Source: CAD feature listing. Evaluate the final solid. Frame: model axes, mm. A direction names the side the tool comes from. Round coordinates to 2 decimals unless told otherwise and drop trailing zeros. Loops run counter-clockwise (first coordinate to the right, second up) from the corner with the lowest first, then second, coordinate; pieces in that order, holes last.
(1) Section A-A, the plane y = 5. Return the cut outline in (x, z), plus the area to 3 significant figures.
(2) Section D-D, the plane y = 38. Return the cut outline in (x, z).
(3) Mould query, pull axis Z, two halves, no side actions, for faces 6 (the flat face through (35, 60, 10)), 7 (the cylindrical face through (62, 12, 0)), 8 (the cylindrical face through (0, 83, -31)). Classes: pulls with the +Z half, pulls with the -Z half, needs draft (parallel to the pull), parting line crosses it, or undercut.
(4) First-contact query: pin 1 Ø5 at (x, y) = (31, 66.5) entering from +Z; pin 2 Ø22 at (x, y) = (-76, 18) entering from +Z; pin 3 Ø13 at (x, z) = (-34.5, 5.5) entering from +Y. Flat tips, straight axial feed; report the tip coordinate or a pass-through.
(5) Set-up query: faces 1 (the flat face through (-80, 12, 8)), 2 (the flat face through (-51.439, 12.325, 37.566)), 3 (the flat face through (80, 12, -8)), 4 (the cylindrical face through (0, 4, 52)), 5 (the flat face through (12, 80, 28)). Return all of +Z, -Z, +X, -X, +Y, -Y with unobstructed straight access to the full face (end or side cutting, diameter ignored); none if empty.
(6) Section C-C, the plane x = 11.5. Return the cut outline in (y, z), plus the area to 3 significant figures.
(7) Section B-B, the plane z = 0. Return the cut outline in (x, y), plus the area to 3 significant figures.
(8) Material intervals for probe 1 along Y at (x, z) = (24, 0); probe 2 along X at (y, z) = (69.5, -4); probe 3 along X at (y, z) = (38.5, 50), sorted ascending.
```python
from build123d import *
from build123d.topology import SkipClean

# Parameters (mm, degrees)
EXTRUDE_1_DEPTH          = 25
SKETCH_2_R               = 45
EXTRUDE_2_DEPTH          = 60
SKETCH_3_R               = 38
CUT_EXTRUDE_1_DEPTH      = 5
SKETCH_4_R               = 24
CUT_EXTRUDE_2_DEPTH      = 132.164019457
CUT_EXTRUDE_3_DEPTH      = 121.016665509
SKETCH_7_W               = 96.437930536
SKETCH_7_H               = 64.787813211
CUT_EXTRUDE_4_DEPTH      = 132.164019457
SKETCH_8_R               = 4
CUT_EXTRUDE_5_DEPTH      = 156.20953579
EXTRUDE_3_REACH          = 158.045
SKETCH_9_R               = 30
CUT_EXTRUDE_6_REACH      = 158.045
CUT_EXTRUDE_6_END_RADIUS = 24
SKETCH_10_R              = 20


with BuildPart() as part:
    # 草图1 → 凸台-拉伸1 (new body)
    with BuildSketch(Plane(origin=(0, 0, 0), x_dir=(1, 0, 0), z_dir=(0, 1, 0))):
        with BuildLine():
            Line((-90, 38), (90, 38))
            Line((90, 38), (90, 8))
            Line((90, 8), (70, 8))
            ThreePointArc((70, 8), (62, 0), (70, -8))
            Line((70, -8), (90, -8))
            Line((90, -8), (90, -25))
            Line((90, -25), (13.942908677, -49.785456613))
            ThreePointArc((13.942908677, -49.785456613), (0, -52), (-13.942908677, -49.785456613))
            Line((-13.942908677, -49.785456613), (-90, -25))
            Line((-90, -25), (-90, -8))
            Line((-90, -8), (-70, -8))
            ThreePointArc((-70, -8), (-62, 0), (-70, 8))
            Line((-70, 8), (-90, 8))
            Line((-90, 8), (-90, 38))
        make_face()
    extrude(amount=EXTRUDE_1_DEPTH)

    # 草图2 → 凸台-拉伸2 (add)
    with SkipClean():  # the faces are left unmerged after this step: merging them gives an invalid solid
        with BuildSketch(Plane(origin=(0, 25, 0), x_dir=(1, 0, 0), z_dir=(0, 1, 0))):
            with Locations(Location((0, -7, 0), (0, 0, 90))):
                Circle(SKETCH_2_R)
        extrude(amount=EXTRUDE_2_DEPTH)

    # 草图3 → 切除-拉伸1 (cut)
    with SkipClean():  # the faces are left unmerged after this step: merging them gives an invalid solid
        with BuildSketch(Plane(origin=(0, 85, 0), x_dir=(1, 0, 0), z_dir=(0, 1, 0))):
            with Locations(Location((0, -7, 0), (0, 0, 270))):
                Circle(SKETCH_3_R)
        extrude(amount=-CUT_EXTRUDE_1_DEPTH, mode=Mode.SUBTRACT)

    # 草图4 → 切除-拉伸2 (cut, through all)
    with SkipClean():  # the faces are left unmerged after this step: merging them gives an invalid solid
        with BuildSketch(Plane(origin=(0, 80, 0), x_dir=(1, 0, 0), z_dir=(0, 1, 0))):
            with Locations(Location((0, -7, 0), (0, 0, 270))):
                Circle(SKETCH_4_R)
        extrude(amount=-CUT_EXTRUDE_2_DEPTH, mode=Mode.SUBTRACT)

    # 草图5 → 切除-拉伸3 (cut, through all)
    with SkipClean():  # the faces are left unmerged after this step: merging them gives an invalid solid
        with BuildSketch(Plane(origin=(0, 60, 0), x_dir=(1, 0, 0), z_dir=(0, 1, 0))):
            with BuildLine():
                Line((-29, 20), (-29, -41.409301068))
                ThreePointArc((-29, -41.409301068), (-44.710463702, -12.096512099), (-36, 20))
                Line((-36, 20), (-29, 20))
            make_face()
            with BuildLine():
                Line((29, 20), (29, -41.409301068))
                ThreePointArc((29, -41.409301068), (44.710463702, -12.096512099), (36, 20))
                Line((36, 20), (29, 20))
            make_face()
        extrude(amount=CUT_EXTRUDE_3_DEPTH, mode=Mode.SUBTRACT)

    # 草图7 → 切除-拉伸4 (cut, through all)
    with SkipClean():  # the faces are left unmerged after this step: merging them gives an invalid solid
        with BuildSketch(Plane(origin=(0, 80, 0), x_dir=(1, 0, 0), z_dir=(0, 1, 0))):
            with Locations((0.609746756, -32.393906605)):
                Rectangle(SKETCH_7_W, SKETCH_7_H)
        extrude(amount=CUT_EXTRUDE_4_DEPTH, mode=Mode.SUBTRACT)

    # 草图8 → 切除-拉伸5 (cut, through all)
    with SkipClean():  # the faces are left unmerged after this step: merging them gives an invalid solid
        with BuildSketch(Plane.ZY.offset(29)):
            with Locations((0, 73)):
                Circle(SKETCH_8_R)
        extrude(amount=-CUT_EXTRUDE_5_DEPTH, mode=Mode.SUBTRACT)

    # 草图9 → 凸台-拉伸3 (add, up to next)
    with BuildSketch(Plane(origin=(0, 0, 57), x_dir=(-1, 0, 0), z_dir=(0, 0, -1)), mode=Mode.PRIVATE) as extrude_3_sk1:
        with Locations(Location((0, 38, 0), (0, 0, 205.679288619))):
            Circle(SKETCH_9_R)
    extrude_3_tool1 = extrude(extrude_3_sk1.sketch, amount=EXTRUDE_3_REACH, mode=Mode.PRIVATE) - part.part
    add(extrude_3_tool1.solids().sort_by_distance((0, 38, 57))[0])

    # 切除-拉伸6: up to this cylinder (the profile starts outside it)
    cut_extrude_6_end = Plane(origin=(0, 38, 7), z_dir=(0, 1, 0)) * Cylinder(CUT_EXTRUDE_6_END_RADIUS, 365.09, mode=Mode.PRIVATE)
    # 草图10 → 切除-拉伸6 (cut, up to the surface)
    with BuildSketch(Plane.XY.offset(57), mode=Mode.PRIVATE) as cut_extrude_6_sk1:
        with Locations((0, 38)):
            Circle(SKETCH_10_R)
    cut_extrude_6_tool1 = extrude(cut_extrude_6_sk1.sketch, amount=-CUT_EXTRUDE_6_REACH, mode=Mode.PRIVATE) - cut_extrude_6_end
    add(cut_extrude_6_tool1.solids().sort_by_distance((0, 38, 57))[0], mode=Mode.SUBTRACT)


solid = part.part
```
Output values:
1. outline: (-90, -38) - (90, -38) - (90, -8) - (70, -8) arc R8 cw to (70, 8) - (90, 8) - (90, 25) - (13.94, 49.79) arc R45 ccw to (-13.94, 49.79) - (-90, 25) - (-90, 8) - (-70, 8) arc R8 cw to (-70, -8) - (-90, -8) - close; hole circle Ø48 at (0, 7)
1. area: 11,300 mm2
2. outline: (-30, 40.54) arc R45 ccw (long way) to (30, 40.54) - (30, 57) - (20, 57) - (20, 20.27) arc R24 cw (long way) to (-20, 20.27) - (-20, 57) - (-30, 57) - close
3. face 6: needs draft
3. face 7: undercut
3. face 8: pulls with the +Z half
4. pin 1: stops at z = 41.82
4. pin 2: stops at z = 33.15
4. pin 3: stops at y = 80
5. face 1: -X, +Y, -Y
5. face 2: +Z, -X, -Y
5. face 3: +X, +Y, -Y
5. face 4: +Z, -Y
5. face 5: +Z, +Y
6. outline: (0, -38) - (25, -38) - (25, -36.51) - (85, -36.51) - (85, -29.22) - (80, -29.22) - (80, -14.07) - (0, -14.07) - close; (0, 28.07) - (21.64, 28.07) - (21.64, 57) - (10.29, 57) - (10.29, 50.51) - (0, 50.51) - close; (54.36, 28.07) - (80, 28.07) - (80, 50.51) - (65.71, 50.51) - (65.71, 57) - (54.36, 57) - close
6. area: 3,080 mm2
7. outline: (-62, 0) - (-22.96, 0) - (-22.96, 69) - (-29, 69) - (-29, 60) - (-44.45, 60) - (-44.45, 25) - (-62, 25) - close; (-29, 77) - (-22.96, 77) - (-22.96, 80) - (-29, 80) - close; (22.96, 0) - (62, 0) - (62, 25) - (44.45, 25) - (44.45, 60) - (29, 60) - (29, 69) - (22.96, 69) - close; (22.96, 77) - (29, 77) - (29, 80) - (22.96, 80) - close
7. area: 3,600 mm2
8. probe 1: y = 0 to 69, 77 to 80
8. probe 2: x = -29 to -21.33, 21.33 to 29
8. probe 3: x = -30 to -19.99, 19.99 to 30
